```python
from build123d import *

# Parameters (mm, degrees)
SKETCH1_W           = 12
SKETCH1_H           = 54.196938457
SKETCH1_H_2         = 12
SKETCH1_W_2         = 21
SKETCH1_H_3         = 19.803061543
BOSS_EXTRUDE1_DEPTH = 4
SKETCH1_3_W         = 12
SKETCH1_3_H         = 54.196938457
SKETCH1_3_H_2       = 19.803061543
SKETCH1_3_H_3       = 12
SKETCH1_3_W_2       = 21
CUT_EXTRUDE3_DEPTH  = 1
SKETCH1_4_W         = 12
SKETCH1_4_H         = 12
CUT_EXTRUDE4_DEPTH  = 2
CHAMFER1_SIZE       = 2
FILLET2_R           = 4
CHAMFER2_SIZE       = 2
CHAMFER2_SIZE2      = 2.383507185
FILLET1_R           = 4
FILLET3_R           = 2
FILLET4_R           = 1
CUT_EXTRUDE6_DEPTH  = 0.5
CUT_EXTRUDE5_DEPTH  = 0.5


with BuildPart() as part:
    # Sketch1 → Boss-Extrude1 (new body)
    with BuildSketch(Plane(origin=(0, 0, 0), x_dir=(1, 0, 0), z_dir=(0, 1, 0))):
        with BuildLine():
            Line((-6, 43), (-6, 44.5))
            Line((-6, 44.5), (-28.5, 44.5))
            Line((-28.5, 44.5), (-28.5, 38))
            ThreePointArc((-28.5, 38), (-16.5, 23.303061543), (-28.5, 8.606123087))
            Line((-28.5, 8.606123087), (-28.5, -11.196938457))
            Line((-28.5, -11.196938457), (-27, -11.196938457))
            Line((-27, -11.196938457), (-6, -11.196938457))
            Line((-6, -11.196938457), (-6, 43))
        make_face()
        with Locations((0, 15.901530771)):
            Rectangle(SKETCH1_W, SKETCH1_H)
        Polygon((27, -44.5), (27, 44.5), (6, 44.5), (6, 43), (6, -11.196938457), (6, -23.196938457), (6, -43), (6, -44.5), align=None)
        with Locations((0, -17.196938457)):
            Rectangle(SKETCH1_W, SKETCH1_H_2)
        with Locations((-16.5, -17.196938457)):
            Rectangle(SKETCH1_W_2, SKETCH1_H_2)
        Polygon((-28.5, -44.5), (-6, -44.5), (-6, -43), (-6, -23.196938457), (-27, -23.196938457), (-28.5, -23.196938457), align=None)
        with Locations((0, -33.098469229)):
            Rectangle(SKETCH1_W, SKETCH1_H_3)
    extrude(amount=BOSS_EXTRUDE1_DEPTH)

    # Sketch1<3> → Cut-Extrude3 (cut)
    with BuildSketch(Plane(origin=(0, 0, 0), x_dir=(1, 0, 0), z_dir=(0, 1, 0))):
        with Locations((0, 15.901530771)):
            Rectangle(SKETCH1_3_W, SKETCH1_3_H)
        with Locations((0, -33.098469229)):
            Rectangle(SKETCH1_3_W, SKETCH1_3_H_2)
        with Locations((0, -17.196938457)):
            Rectangle(SKETCH1_3_W, SKETCH1_3_H_3)
        with Locations((-16.5, -17.196938457)):
            Rectangle(SKETCH1_3_W_2, SKETCH1_3_H_3)
    extrude(amount=CUT_EXTRUDE3_DEPTH, mode=Mode.SUBTRACT)

    # Sketch1<4> → Cut-Extrude4 (cut)
    with BuildSketch(Plane(origin=(0, 0, 0), x_dir=(1, 0, 0), z_dir=(0, 1, 0))):
        with Locations((0, -17.196938457)):
            Rectangle(SKETCH1_4_W, SKETCH1_4_H)
    extrude(amount=CUT_EXTRUDE4_DEPTH, mode=Mode.SUBTRACT)

    # Chamfer1
    # the kernel refuses this chamfer: 2 mm, written as the material it takes off along each edge
    with BuildSketch(Plane(origin=(-6, 1, 23.196938457), x_dir=(0, 1, 0), z_dir=(0, 0, -1))) as chamfer1_piece_1_section:
        Polygon((CHAMFER1_SIZE, 0), (0, -CHAMFER1_SIZE), (0, 0), align=None)
    chamfer1_piece_1 = extrude(amount=12, mode=Mode.PRIVATE)
    chamfer1_piece_1 = split(chamfer1_piece_1, bisect_by=Plane(origin=(-6, 2, 23.196938457), z_dir=(0, -1, 0)), keep=Keep.TOP, mode=Mode.PRIVATE)
    add(chamfer1_piece_1, mode=Mode.SUBTRACT)

    # Fillet2
    fillet2_edges = [part.edges().sort_by_distance(p)[0] for p in [
        (-28.5, 2, -8.606123087),
        (-28.5, 2, -38),
    ]]
    fillet(fillet2_edges, radius=FILLET2_R)

    # Chamfer2
    chamfer2_edges = [part.edges().sort_by_distance(p)[0] for p in [
        (27, 4, 0),
    ]]
    chamfer2_side = [part.faces().sort_by_distance(p)[0] for p in [
        (0.667186488, 4, 1.280693721),
    ]]
    chamfer(chamfer2_edges, length=CHAMFER2_SIZE, length2=CHAMFER2_SIZE2, reference=chamfer2_side[0])

    # Fillet1
    # the kernel refuses this fillet: 4 mm, written as the material it takes off along each edge
    with BuildSketch(Plane(origin=(-28.5, -10, 44.5), x_dir=(1, 0, 0), z_dir=(0, 1, 0))) as fillet1_piece_1:
        with BuildLine():
            CenterArc((FILLET1_R, FILLET1_R), FILLET1_R, 180, 90)
            Line((0, FILLET1_R), (-FILLET1_R * 0.02, FILLET1_R))
            Line((-FILLET1_R * 0.02, FILLET1_R), (-FILLET1_R * 0.02, -FILLET1_R * 0.02))
            Line((-FILLET1_R * 0.02, -FILLET1_R * 0.02), (FILLET1_R, -FILLET1_R * 0.02))
            Line((FILLET1_R, -FILLET1_R * 0.02), (FILLET1_R, 0))
        make_face()
    extrude(amount=24, mode=Mode.SUBTRACT)
    with BuildSketch(Plane(origin=(-28.5, -9.931735764, -44.5), x_dir=(1, 0, 0), z_dir=(0, 1, 0))) as fillet1_piece_2:
        with BuildLine():
            CenterArc((3.972694306, -4), FILLET1_R, 90, 83.301437518)
            Line((0, -3.533416724), (-0.079453886, -3.524085059))
            ThreePointArc((-0.079453886, -3.524085059), (-0.08, -1.766708362), (-0.08, 0))
            Line((-0.08, 0), (0, 0.08))
            Line((0, 0.08), (3.972694306, 0.08))
            Line((3.972694306, 0.08), (3.972694306, 0))
        make_face()
    extrude(amount=23.863471529, mode=Mode.SUBTRACT)
    with BuildSketch(Plane(origin=(27, -10, -44.5), x_dir=(-1, 0, 0), z_dir=(0, 1, 0))) as fillet1_piece_3:
        with BuildLine():
            CenterArc((FILLET1_R, FILLET1_R), FILLET1_R, 180, 90)
            Line((0, FILLET1_R), (-FILLET1_R * 0.02, FILLET1_R))
            Line((-FILLET1_R * 0.02, FILLET1_R), (-FILLET1_R * 0.02, -FILLET1_R * 0.02))
            Line((-FILLET1_R * 0.02, -FILLET1_R * 0.02), (FILLET1_R, -FILLET1_R * 0.02))
            Line((FILLET1_R, -FILLET1_R * 0.02), (FILLET1_R, 0))
        make_face()
    extrude(amount=21.616492815, mode=Mode.SUBTRACT)
    with BuildSketch(Plane(origin=(27, -10, 44.5), x_dir=(-1, 0, 0), z_dir=(0, 1, 0))) as fillet1_piece_4:
        with BuildLine():
            CenterArc((FILLET1_R, -FILLET1_R), FILLET1_R, 90, 90)
            Line((0, -FILLET1_R), (-FILLET1_R * 0.02, -FILLET1_R))
            Line((-FILLET1_R * 0.02, -FILLET1_R), (-FILLET1_R * 0.02, FILLET1_R * 0.02))
            Line((-FILLET1_R * 0.02, FILLET1_R * 0.02), (FILLET1_R, FILLET1_R * 0.02))
            Line((FILLET1_R, FILLET1_R * 0.02), (FILLET1_R, 0))
        make_face()
    extrude(amount=21.616492815, mode=Mode.SUBTRACT)

    # Fillet3
    fillet3_edges = [part.edges().sort_by_distance(p)[0] for p in [
        (0, 1, -43),
        (0, 1, 43),
    ]]
    fillet(fillet3_edges, radius=FILLET3_R)

    # Fillet4
    fillet4_edges = [part.edges().sort_by_distance(p)[0] for p in [
        (-6, 2, 44.5),
        (-28.5, 2, 23.196938457),
        (-28.5, 2, 11.196938457),
        (-6, 2, -44.5),
        (6, 2, -44.5),
        (6, 2, 44.5),
    ]]
    fillet(fillet4_edges, radius=FILLET4_R)

    # Sketch3 → Cut-Extrude6 (cut)
    with BuildSketch(Plane.XZ):
        Polygon((26, 6.846975509), (26, -2.047005384), (22.5, -0.026279442), (22.5, 7.713000913), (18.5, 10.022401989), (18.5, 2.283121635), (16.5, 3.437822174), (16.5, 12.331803066), align=None)
        Polygon((9, 7.767949192), (9, 18.971331162), (26, 9.156376586), (26, 12.620478201), (9, 22.435432777), (9, 25.855728078), (13.872673559, 23.042488687), (13.872673559, 33.014498231), (11.872673559, 34.16919877), (11.872673559, 25.351889764), (7, 28.165129155), (7, 8.922649731), align=None)
        Polygon((14.5, 4.592522712), (11, 6.613248654), (11, 15.507229547), (14.5, 13.486503605), align=None)
        Polygon((26, 19.084579816), (21.241040405, 21.832166419), (21.241040405, 18.832166419), (26, 16.084579816), align=None)
        Polygon((18.5, 26.87880845), (18.5, 19.260006297), (16.5, 20.414706835), (16.5, 31.497610604), (26, 26.012783046), (26, 22.548681431), align=None)
        Polygon((26, 34.095686815), (26, 28.322184123), (9, 38.137138699), (9, 29.742507874), (7, 30.897208412), (7, 40.446539776), (22.5, 31.497610604), (22.5, 34.961712219), (13.872673559, 39.942701462), (13.872673559, 43.5), (15.872673559, 43.5), (15.872673559, 39.942701462), align=None)
        Polygon((26, 36.405087892), (18.855212659, 40.530132787), (18.855212659, 43.5), (22.355212659, 43.5), (22.355212659, 39.664107383), (26, 37.55978843), align=None)
        Polygon((12.038363906, 41.001740633), (7.711251753, 43.5), (12.038363906, 43.5), align=None)
    extrude(amount=-CUT_EXTRUDE6_DEPTH, mode=Mode.SUBTRACT)

    # Sketch2 → Cut-Extrude5 (cut)
    # profile 1 of 3: a face of its own
    with BuildSketch(Plane.XZ):
        with BuildLine():
            Line((21.258663757, -19.559912495), (21.258663757, -31.236746335))
            ThreePointArc((21.258663757, -31.236746335), (16.804977927, -25.398329415), (21.258663757, -19.559912495))
        make_face()
        with BuildLine():
            ThreePointArc((20.558663757, -20.563874743), (17.504977927, -25.398329415), (20.558663757, -30.232784086))
            Line((20.558663757, -30.232784086), (20.558663757, -28.325034046))
            Line((20.558663757, -28.325034046), (20.558663757, -22.471624783))
            Line((20.558663757, -22.471624783), (20.558663757, -20.563874743))
        make_face(mode=Mode.SUBTRACT)
    # profile 2 of 3: a face of its own
    with BuildSketch(Plane.XZ):
        with BuildLine():
            Line((20.558663757, -22.471624783), (20.558663757, -28.325034046))
            ThreePointArc((20.558663757, -28.325034046), (18.838663757, -25.398329415), (20.558663757, -22.471624783))
        make_face()
    # profile 3 of 3: a face of its own
    with BuildSketch(Plane.XZ):
        with BuildLine():
            ThreePointArc((20.075747841, -19.354579409), (16.204977927, -25.398329415), (20.075747841, -31.442079421))
            ThreePointArc((20.075747841, -31.442079421), (20.402353273, -32.080361375), (19.859139802, -32.548329415))
            Line((19.859139802, -32.548329415), (11.741336243, -32.548329415))
            Line((11.741336243, -32.548329415), (11.741336243, -31.348329415))
            Line((11.741336243, -31.348329415), (17.887029825, -31.348329415))
            ThreePointArc((17.887029825, -31.348329415), (16.002102254, -29.018717282), (15.141336243, -26.148329415))
            Line((15.141336243, -26.148329415), (11.741336243, -26.148329415))
            Line((11.741336243, -26.148329415), (11.741336243, -24.648329415))
            Line((11.741336243, -24.648329415), (15.141336243, -24.648329415))
            ThreePointArc((15.141336243, -24.648329415), (16.002102254, -21.777941547), (17.887029825, -19.448329415))
            Line((17.887029825, -19.448329415), (11.741336243, -19.448329415))
            Line((11.741336243, -19.448329415), (11.741336243, -18.248329415))
            Line((11.741336243, -18.248329415), (19.859139802, -18.248329415))
            ThreePointArc((19.859139802, -18.248329415), (20.402353273, -18.716297455), (20.075747841, -19.354579409))
        make_face()
    extrude(amount=-CUT_EXTRUDE5_DEPTH, mode=Mode.SUBTRACT)


solid = part.part
```
Build history of the part. All positions in model axes, mm. A direction names the side the tool comes from. Round coordinates to 2 decimals unless told otherwise and drop trailing zeros. Order: outer loops, then holes, each group sorted by start corner. A loop starts at its lowest first (then second) coordinate and runs counter-clockwise, first axis right, second up. Notation, with made-up numbers: (47, 50.5) - (88, 50.5) arc R14 cw to (88, 57.5) - close; hole circle Ø8 at (-12.75, 8.5). An arc over 180 degrees is marked (long way). Use a Markdown table: item, result.
1) Saw through at B-B on x = 5. Write the cut outline in (y, z).
Recorded:
| item | result |
|---|---|
| outline | (1, -41) arc R2 ccw to (3, -43) - (4, -43) - (4, 43) - (3, 43) arc R2 ccw to (1, 41) - (1, 23.2) - (2, 23.2) - (2, 11.2) - (1, 11.2) - close |
2) Wall check: L1, parallel to X at y = 0.65, z = 34; L2, parallel to X at y = 0.3, z = -19; L3, parallel to Y at x = -4.5, z = -39.5. Give the ranges that are in metal, low to high.
Recorded:
| item | result |
|---|---|
| L1 | x = -28.5 to -6, 6 to 27 |
| L2 | x = -17.13 to -6, 6 to 11.74, 20.39 to 27 |
| L3 | y = 1 to 4 |
3) Saw through at A-A on x = -20. Write the cut outline in (y, z), and give its area (3 significant figures).
Recorded:
| item | result |
|---|---|
| outline | (0, -44.5) - (4, -44.5) - (4, -32.93) - (0, -32.93) - close; (0, -13.67) - (4, -13.67) - (4, 44.5) - (0, 44.5) - (0, 23.2) - (1, 23.2) - (1, 11.2) - (0, 11.2) - close |
| area | 267 mm² |
4) Pull direction X, two halves, no side cores. Call faces 1 (the face through (18.67, 0, -25.47)), 2 (the face through (22, 0.5, 40)), 3 (the face through (25.26, 1.53, 43.8)), 4 (the face through (-28.5, 2, 2)): pulls with the +X half, pulls with the -X half, needs draft (parallel to the pull), parting line crosses it, or undercut.
Recorded:
| item | result |
|---|---|
| face 1 | needs draft |
| face 2 | undercut |
| face 3 | pulls with the +X half |
| face 4 | pulls with the -X half |
5) Saw through at C-C on z = -11. Write the cut outline in (x, y), and give its area (3 significant figures).
Recorded:
| item | result |
|---|---|
| outline | (-22.92, 0) - (-6, 0) - (-6, 1) - (6, 1) - (6, 0) - (27, 0) - (27, 1.62) - (25, 4) - (-22.92, 4) - close |
| area | 185 mm² |
6) Flat gauge pins, fed straight in: pin 1 Ø1.2 at (y, z) = (3, 12.5) entering from -X; pin 2 Ø0.8 at (x, y) = (0, 3.5) entering from -Z; pin 3 Ø0.6 at (y, z) = (0.5, 43) entering from -X. Where does each tip first touch, or does it go through?
Recorded:
| item | result |
|---|---|
| pin 1 | stops at x = -27 |
| pin 2 | stops at z = -43 |
| pin 3 | stops at x = -27.84 |
7) Tool access for faces 5 (the face through (16.022, 0.246, -29.056)), 6 (the face through (-27.8, 2, -7.9)), 7 (the face through (16, 0, -11)), 8 (the face through (0.08, 1.6, 42.43)): list every direction of +Z, -Z, +X, -X, +Y, -Y with a clear straight run to the whole face (end or side of a thin tool).
Recorded:
| item | result |
|---|---|
| face 5 | -Y |
| face 6 | -X, +Y, -Y |
| face 7 | +Z, -Z, +X, -X, -Y |
| face 8 | +Z, -Y |
